```python
from build123d import *

# Parameters (mm, degrees)
F1_W     = 14.6656349089
F1_H     = 0.1217532289
F2_ANGLE = 20


with BuildPart() as f2:
    # F1 (on Front) → F2 (revolve)
    with BuildSketch(Plane.XZ):
        Polygon((-43.7767438772, 12.7751471548), (-43.8843175875, 12.7008123937), (-43.7714494091, 12.7659768669), align=None)
        Polygon((-36.4386319546, 0.0651644732), (-36.5515001331, 0), (-36.4439264228, -0.0621077106), (-36.3309057177, -0.1273602451), (-34.3620503103, -1.2640794445), (-34.3620503103, 1.2640794445), align=None)
        Polygon((-58.7149140006, 12.7960529626), (-58.5499524964, 12.7008123937), (-58.5499524964, 12.8391478211), (-58.5499524964, 15.2491778135), (-60.7598529608, 13.9766990217), align=None)
        Polygon((-43.7767438772, -12.7629201043), (-43.8843175875, -12.7008123937), (-43.8843175875, -12.8225656226), (-43.8843175875, -15.2283469215), (-41.6742515512, -13.9767946147), align=None)
        Polygon((-58.5499524964, -12.8225656226), (-58.5499524964, -12.7008123937), (-58.6575262067, -12.7629201043), (-60.7503676631, -13.9712226825), (-58.5499524964, -15.2283469215), align=None)
        Polygon((-65.9903436611, -0.0621077106), (-65.8827699508, 0), (-65.9900653034, 0.0619470007), (-68.0832503253, 1.2704479365), (-68.0832503253, -1.2704479365), align=None)
        Polygon((-43.8843175875, 12.7008123937), (-36.5515001331, 0), (-36.4386319546, 0.0651644732), (-43.7714494091, 12.7659768669), align=None)
        Polygon((-36.5515001331, 0), (-43.8843175875, -12.7008123937), (-43.7767438772, -12.7629201043), (-36.4439264228, -0.0621077106), align=None)
        Polygon((-58.5499524964, 12.8391478211), (-58.5499524964, 12.7008123937), (-51.217135042, 12.7008123937), (-43.8843175875, 12.7008123937), (-43.8843175875, 12.8391478211), align=None)
        Polygon((-43.8843175875, 15.2525296435), (-43.8843175875, 12.8391478211), (-43.8843175875, 12.7008123937), (-43.7767438772, 12.7751471548), (-43.7714494091, 12.7659768669), (-41.6910577545, 13.9670915487), align=None)
        Polygon((-65.9900653034, 0.0619470007), (-65.8827699508, 0), (-58.5499524964, 12.7008123937), (-58.7149140006, 12.7960529626), align=None)
        with Locations((-51.217135042, -12.7616890082)):
            Rectangle(F1_W, F1_H)
        Polygon((-58.5499524964, -12.7008123937), (-65.8827699508, 0), (-65.9903436611, -0.0621077106), (-65.9526700928, -0.1273602451), (-58.6575262067, -12.7629201043), align=None)
    revolve(axis=Axis((0, 0, 0), (0, 0, 1)), revolution_arc=F2_ANGLE)


solid = f2.part
```
The model under review builds one solid part; all positions refer to its coordinate system, in mm. A direction names the side the tool comes from. Round coordinates to 2 decimals unless told otherwise and drop trailing zeros. Order: outer loops, then holes, each group sorted by start corner. A loop starts at its lowest first (then second) coordinate and runs counter-clockwise, first axis right, second up. Notation, with made-up numbers: (51, -38.75) -> (99, -38.75) arc R28 cw to (99, -12.75) -> close; hole circle Ø8 at (55, 18.5). An arc over 180 degrees is marked (long way). One line per item, written item: value. Start each with the question number.
Q1. Machinability: for faces 5 (the face through (-41.931, -7.288, 14.476)), 6 (the face through (-58.547, -10.176, 14.745)), 7 (the face through (-65.83, -11.44, 0.54)), 8 (the face through (-41.879, -7.279, -13.496)), 9 (the face through (-58.607, -10.186, -13.241)), which of the approach directions +Z, -Z, +X, -X, +Y, -Y give a long, thin tool a straight path to every point of the face, cutting with its end or side? Answer none if there is none.
Q2. Clearance check with flat-ended pins moving along their axes: pin 1 Ø2 at (x, y) = (-38.5, -15.5) entering from +Z; pin 2 Ø1 at (x, y) = (-55.5, -4.5) entering from +Z; pin 3 Ø1 at (x, y) = (-58.5, -9) entering from -Z; pin 4 Ø2 at (y, z) = (-7, -5) entering from +X. State where each tip first meets the part, or that it passes through.
Q3. Take a section at B-B (z = -7). Write out the cut boundary in (x, y).
Q4. Mouldability with a two-part tool opening along Y and no side actions: class faces 1 (the face through (-65.8, -11.44, -0.52)), 2 (the face through (-43.236, -7.515, 14.029)), 3 (the face through (-34.664, -6.025, 0.789)), 4 (the face through (-61.247, -10.645, 6.439)) as released by +Y, released by -Y, zero draft, split by the parting line, or undercut.
Q5. Wall thickness on line 1 (X direction, y = -14.25, z = 10); line 2 (X direction, y = -11.75, z = -13); line 3 (X direction, y = -18.75, z = -3.5): over which ranges is each line inside the solid? List them lowest first.
Q6. Take a section at A-A (x = -51.5). Write out the cut boundary in (y, z), and give its area (3 significant figures).
Reported:
1. face 5: +Z, +X, +Y
1. face 6: +Z, -X, -Y
1. face 7: +Z
1. face 8: +X, +Y
1. face 9: -X, -Y
2. pin 1: passes through
2. pin 2: stops at z = 12.84
2. pin 3: stops at z = -15.15
2. pin 4: stops at x = -38.05
3. outline: (-61.98, 0) arc R61.98 ccw to (-58.25, -21.2) -> (-58.11, -21.15) arc R61.84 cw to (-61.84, 0) -> close; (-40.59, 0) arc R40.59 ccw to (-38.14, -13.88) -> (-38.01, -13.83) arc R40.45 cw to (-40.45, 0) -> close
4. face 1: undercut
4. face 2: released by -Y
4. face 3: undercut
4. face 4: released by +Y
5. line 1: x = -58.6 to -58.4, -39.85 to -39.69
5. line 2: x = -57.89 to -57.36, -42.28 to -41.74
5. line 3: x = -61.2 to -61.05
6. outline: (-18.74, -12.82) -> (0, -12.82) -> (0, -12.7) -> (-18.74, -12.7) -> close; (-18.74, 12.7) -> (0, 12.7) -> (0, 12.84) -> (-18.74, 12.84) -> close
6. area: 4.88 mm2
